from build123d import *

# Parameters (mm, degrees)
SKETCH1_W           = 30
SKETCH1_H           = 16
BOSS_EXTRUDE1_DEPTH = 30
CUT_EXTRUDE1_REACH  = 47.343
SKETCH2_R           = 2.1
SKETCH3_R           = 4
CUT_EXTRUDE2_DEPTH  = 6.5
SKETCH4_R           = 3.5
CUT_EXTRUDE3_DEPTH  = 14
SKETCH6_W           = 6.374381548
SKETCH6_H           = 2.3
CUT_EXTRUDE8_DEPTH  = 46.343136195
SKETCH7_R           = 1.5
CUT_EXTRUDE9_DEPTH  = 8


with BuildPart() as part:
    # Sketch1 → Boss-Extrude1 (new body)
    with BuildSketch(Plane(origin=(0, 0, 0), x_dir=(1, 0, 0), z_dir=(0, 1, 0))):
        with Locations((15, 8)):
            Rectangle(SKETCH1_W, SKETCH1_H)
    extrude(amount=BOSS_EXTRUDE1_DEPTH)

    # Sketch2 → Cut-Extrude1 (cut, up to next)
    with BuildSketch(Plane(origin=(0, 30, 0), x_dir=(1, 0, 0), z_dir=(0, 1, 0)), mode=Mode.PRIVATE) as cut_extrude1_sk1:
        with Locations(Location((6.5, 6, 0), (0, 0, 270))):
            Circle(SKETCH2_R)
    cut_extrude1_tool1 = extrude(cut_extrude1_sk1.sketch, amount=-CUT_EXTRUDE1_REACH, mode=Mode.PRIVATE) & part.part
    # Sketch2 → Cut-Extrude1 (cut, up to next)
    with BuildSketch(Plane(origin=(0, 30, 0), x_dir=(1, 0, 0), z_dir=(0, 1, 0)), mode=Mode.PRIVATE) as cut_extrude1_sk2:
        with Locations(Location((23.5, 6, 0), (0, 0, 270))):
            Circle(SKETCH2_R)
    cut_extrude1_tool2 = extrude(cut_extrude1_sk2.sketch, amount=-CUT_EXTRUDE1_REACH, mode=Mode.PRIVATE) & part.part
    add(cut_extrude1_tool1.solids().sort_by_distance((6.5, 30, -6))[0], mode=Mode.SUBTRACT)
    add(cut_extrude1_tool2.solids().sort_by_distance((23.5, 30, -6))[0], mode=Mode.SUBTRACT)

    # Sketch3 → Cut-Extrude2 (cut)
    with BuildSketch(Plane(origin=(0, 30, 0), x_dir=(1, 0, 0), z_dir=(0, 1, 0))):
        with Locations(Location((6.5, 6, 0), (0, 0, 270))):
            Circle(SKETCH3_R)
        with Locations(Location((23.5, 6, 0), (0, 0, 270))):
            Circle(SKETCH3_R)
    extrude(amount=-CUT_EXTRUDE2_DEPTH, mode=Mode.SUBTRACT)

    # Sketch4 → Cut-Extrude3 (cut)
    with BuildSketch(Plane.XZ):
        with Locations(Location((6.5, -6, 0), (0, 0, 270))):
            Circle(SKETCH4_R)
        with Locations(Location((23.5, -6, 0), (0, 0, 270))):
            Circle(SKETCH4_R)
    extrude(amount=-CUT_EXTRUDE3_DEPTH, mode=Mode.SUBTRACT)

    # Sketch6 → Cut-Extrude8 (cut, through all)
    with BuildSketch(Plane(origin=(30, 0, 0), x_dir=(0, 0, -1), z_dir=(1, 0, 0))):
        with Locations((14.187190774, 2.4)):
            Rectangle(SKETCH6_W, SKETCH6_H)
        with Locations((14.187190774, 6.65)):
            Rectangle(SKETCH6_W, SKETCH6_H)
        with Locations((14.187190774, 10.9)):
            Rectangle(SKETCH6_W, SKETCH6_H)
        with Locations((14.187190774, 15.15)):
            Rectangle(SKETCH6_W, SKETCH6_H)
        with Locations((14.187190774, 19.4)):
            Rectangle(SKETCH6_W, SKETCH6_H)
        with Locations((14.187190774, 23.65)):
            Rectangle(SKETCH6_W, SKETCH6_H)
        with Locations((14.187190774, 27.9)):
            Rectangle(SKETCH6_W, SKETCH6_H)
    extrude(amount=-CUT_EXTRUDE8_DEPTH, mode=Mode.SUBTRACT)

    # Sketch7 → Cut-Extrude9 (cut)
    with BuildSketch(Plane.XY):
        with Locations((15, 10)):
            Circle(SKETCH7_R)
        with Locations((10.5, 20)):
            Circle(SKETCH7_R)
        with Locations((19.5, 20)):
            Circle(SKETCH7_R)
    extrude(amount=-CUT_EXTRUDE9_DEPTH, mode=Mode.SUBTRACT)


solid = part.part
Source: CAD feature listing. Evaluate the final solid. Frame: model axes, mm. A direction names the side the tool comes from. Give positions to 0.01 mm unless a question says otherwise; leave off trailing zeros. Write each loop counter-clockwise with the first axis right and the second up, starting at its lowest first coordinate (ties: lowest second). Pieces come first, ordered by that corner, then holes. Notation, with made-up numbers: (46, 19.5) - (100, 19.5) arc R33 ccw to (100, 48.5) - close; hole circle Ø11 at (37.5, 30.5). An arc over 180 degrees is marked (long way). Write item = value, one per line. Start each with the question number.
Q1. Reachability of faces 4 (the flat face through (15, 15, -11)), 5 (the flat face through (22, 14, -8)), 6 (the cylindrical face through (2.595, 26.796, -6.867)) from +Z, -Z, +X, -X, +Y, -Y: full face, straight path, thin tool, end or side. Return the list, or none.
Q2. Material intervals for probe 1 along X at (y, z) = (18.25, -6); probe 2 along X at (y, z) = (26.75, -6); probe 3 along Z at (x, y) = (11, 28.75), sorted ascending.
Q3. Cut plane D-D, the plane y = 26.25. Return loops of the section in (x, z), then the cut area to 3 significant figures.
Q4. Pin query (flat end, axial travel): pin 1 Ø1.5 at (x, y) = (19, 19.5) entering from +Z; pin 2 Ø3.5 at (x, z) = (23.5, -6) entering from +Y; pin 3 Ø3.5 at (x, z) = (24, -5) entering from -Y; pin 4 Ø0.7 at (x, y) = (9.5, 15) entering from -Z. Return the tip coordinate at first contact, or that it passes through.
Q5. Cut plane A-A, the plane z = -6. Give the number of separate pieces and of enclosed holes in the cut face, then the cut area to 3 significant figures.
Q6. Cut plane C-C, the plane y = 20. Return loops of the section in (x, z), then the cut area to 3 significant figures.
Q7. Draft query along X for faces 1 (the flat face through (15, 5.5, -13)), 2 (the flat face through (30, 15, -6)), 3 (the flat face through (10, 20, -8)). Return one class per face: +X half, -X half, draft (parallel to the pull), parting line (faces both ways), or undercut.
Computed values:
q1.face_4 = -Z, +X, -X
q1.face_5 = -Y
q1.face_6 = +Y
q2.probe_1 = 0 to 4.4, 8.6 to 21.4, 25.6 to 30
q2.probe_2 = 0 to 2.5, 10.5 to 19.5, 27.5 to 30
q2.probe_3 = -11 to 0
q3.outline = (0, -16) - (30, -16) - (30, 0) - (0, 0) - close; hole circle Ø8 at (6.5, -6); hole circle Ø8 at (23.5, -6)
q3.area = 379 mm²
q4.pin_1 = -8
q4.pin_2 = through
q4.pin_3 = 14
q4.pin_4 = -11
q5.separate_pieces = 3
q5.enclosed_holes = 3
q5.area = 499 mm²
q6.outline = (0, -11) - (30, -11) - (30, 0) - (21, 0) - (21, -8) - (18, -8) - (18, 0) - (12, 0) - (12, -8) - (9, -8) - (9, 0) - (0, 0) - close; hole circle Ø4.2 at (6.5, -6); hole circle Ø4.2 at (23.5, -6)
q6.area = 254 mm²
q7.face_1 = draft
q7.face_2 = +X half
q7.face_3 = undercut
